Could you check a few things on this model? Use its own coordinates, in mm. A direction names the side the tool comes from. Give positions to 0.01 mm unless a question says otherwise; leave off trailing zeros. Loops run counter-clockwise (first coordinate to the right, second up) from the corner with the lowest first, then second, coordinate; pieces in that order, holes last. Notation, with made-up numbers: (79, -34.5) -> (136, -34.5) arc R28 ccw to (136, -4.5) -> close; hole circle Ø1 at (23, 62). An arc over 180 degrees is marked (long way). Put each result on its own line as item: value.
```python
from build123d import *

# Parameters (mm, degrees)
F4_DEPTH = 1.25
F5_R     = 0.5


with BuildPart() as f1:
    # F0 (on Front) → F1 (revolve)
    with BuildSketch(Plane.XZ):
        Polygon((1.5, 16), (0, 16), (0, -2.5), (2.93934, -2.5), (4, -1.43934), (4, 0), (1.5, 0), align=None)
    revolve(axis=Axis((0, 0, 6.75), (0, 0, -1)))

    # F3 (on offset) → F4 (join, symmetric)
    with BuildSketch(Plane.XY.offset(10)):
        Polygon((3, -1.732051), (3, 1.732051), (0, 3.464102), (-3, 1.732051), (-3, -1.732051), (0, -3.464102), align=None)
    extrude(amount=F4_DEPTH, both=True)

    # F5
    f5_edges = [f1.edges().sort_by_distance(p)[0] for p in [
        (1.5, -2.598076, 11.25),
        (3, 0, 11.25),
        (1.5, 2.598076, 11.25),
        (-1.5, -2.598076, 11.25),
        (-3, 0, 11.25),
        (-1.5, 2.598076, 11.25),
        (-1.5, -2.598076, 8.75),
        (1.5, -2.598076, 8.75),
        (3, 0, 8.75),
        (-3, 0, 8.75),
        (-1.5, 2.598076, 8.75),
        (1.5, 2.598076, 8.75),
    ]]
    fillet(f5_edges, radius=F5_R)


solid = f1.part
```
1. For faces 4 (the face through (-1.4, -2.48, 8.89)), 5 (the face through (-1.15, -1.24, 11.25)), 6 (the face through (-1.446, 2.456, 8.893)), 7 (the face through (1.5, -2.6, 10)), which set-ups out of +Z, -Z, +X, -X, +Y, -Y let a thin tool reach every point of the face, with its end or its side?
Recorded:
face 4: -X, -Y
face 5: +Z
face 6: -X, +Y
face 7: +Z, +X, -Y
2. If we section it at C-C (z = -0.75): List the corners of the cut face in (x, y) for me, then the cut area to 3 significant figures.
Recorded:
outline: circle Ø8 at (0, 0)
area: 50.3 mm^2
3. I need wall thicknesses on line 1 (Z direction, x = 0.5, y = -2.5); line 2 (X direction, y = -2, z = -0.75); line 3 (X direction, y = -0.75, z = 10.5). Which ranges of each line are inside material? Lowest first, please.
Recorded:
line 1: z = -2.5 to 0, 8.75 to 11.25
line 2: x = -3.46 to 3.46
line 3: x = -3 to 3
4. Thinking about a two-plate mould opening in Z: for faces 1 (the face through (-1.4, -2.48, 11.11)), 2 (the face through (2, 0, 0)), 3 (the face through (3, 0, 10)), which applies, pulls with the +Z half, pulls with the -Z half, needs draft (parallel to the pull), parting line crosses it, or undercut?
Recorded:
face 1: pulls with the +Z half
face 2: undercut
face 3: needs draft
5. I'm going to push flat-ended pins straight in: pin 1 (2 mm diameter, centred on x = -2, y = 2.5, fed in from -Z); pin 2 (1.5 mm diameter, centred on y = 2, z = 9.5, fed in from -X); pin 3 (1.2 mm diameter, centred on y = -1, z = 10, fed in from +X); pin 4 (2 mm diameter, centred on x = 2, z = 4.5, fed in from -Y). Where does each tip first touch, or does it pass through?
Recorded:
pin 1: stops at z = -2.5
pin 2: stops at x = -3
pin 3: stops at x = 3
pin 4: stops at y = -1.12
6. If we section it at B-B (z = 2.5): List the corners of the cut face in (x, y) for me, then the cut area to 3 significant figures.
Recorded:
outline: circle Ø3 at (0, 0)
area: 7.07 mm^2
7. If we section it at A-A (y = 0): List the corners of the cut face in (x, z) for me.
Recorded:
outline: (-4, -1.44) -> (-2.94, -2.5) -> (2.94, -2.5) -> (4, -1.44) -> (4, 0) -> (1.5, 0) -> (1.5, 8.75) -> (2.5, 8.75) arc R0.5 ccw to (3, 9.25) -> (3, 10.75) arc R0.5 ccw to (2.5, 11.25) -> (1.5, 11.25) -> (1.5, 16) -> (-1.5, 16) -> (-1.5, 11.25) -> (-2.5, 11.25) arc R0.5 ccw to (-3, 10.75) -> (-3, 9.25) arc R0.5 ccw to (-2.5, 8.75) -> (-1.5, 8.75) -> (-1.5, 0) -> (-4, 0) -> close
